from build123d import *

# Parameters (mm, degrees)
F1_FACE_R   = 15
F1_FACE_R_2 = 7
F2_DEPTH    = 5
F4_DEPTH    = 20


with BuildPart() as f1:
    # F0 (on Front) → F1 (revolve)
    with BuildSketch(Plane.XZ):
        Polygon((7, 27), (4, 27), (4, 8), (3, 8), (3, 4.470672), (4, 3.561659), (4, 0), (4, -1), (0, -1), (0, -25), (15, -25), (15, 27), (15, 30), (7, 30), align=None)
    revolve(axis=Axis((0, 0, -12.5), (0, 0, 1)))

    # F1_face (on face) → F2 (join)
    with BuildSketch(Plane.XY.offset(30)):
        Circle(F1_FACE_R)
        Circle(F1_FACE_R_2, mode=Mode.SUBTRACT)
    extrude(amount=F2_DEPTH)

    # F3 (on Front) → F4 (cut, symmetric)
    with BuildSketch(Plane.XZ):
        with BuildLine():
            Line((10.994077, 35.048041), (-10.997782, 35.048041))
            ThreePointArc((-10.997782, 35.048041), (-0.001852, 30), (10.994077, 35.048041))
        make_face()
    extrude(amount=F4_DEPTH, both=True, mode=Mode.SUBTRACT)


solid = f1.part
Work out the finished part from the listing and answer in its coordinate system (mm). A direction names the side the tool comes from. Coordinates: 2 decimals unless noted, no trailing zeros. Loops run counter-clockwise (first coordinate to the right, second up) from the corner with the lowest first, then second, coordinate; pieces in that order, holes last. Notation, with made-up numbers: M 52.5,89 L 70.5,89 A22 cw 70.5,118 Z; hole C 15,52.25 d10. An arc over 180 degrees is marked long. Answer in a Markdown table with one row per item. Add a question column.
1. Find section B-B, the plane x = 6. Write down the section's boundary in (y, z), then the cut area to 3 significant figures.
2. Find section C-C, the plane y = 5. Write down the section's boundary in (x, z).
3. Find section D-D, the plane z = -4. Write down the section's boundary in (x, y), then the cut area to 3 significant figures.
4. Consider L1, parallel to Y at x = 0, z = 1.1; L2, parallel to X at y = 0, z = 28.8; L3, parallel to Z at x = -6.5, y = -1.5. Determine where each line is inside the solid, lowest interval first.
5. Find section A-A, the plane z = 29. Write down the section's boundary in (x, y).
6. A tool of negligible diameter and unlimited length cuts with its end or side. For faces 1 (the cylindrical face through (-2.915, -6.877, 30.296)), 2 (the flat face through (3, -3, 27)), 3 (the cylindrical face through (-0.867, -3.905, 1.249)), from which of +Z, -Z, +X, -X, +Y, -Y can it reach the whole face along a straight path? Write none if from no direction.
7. The mould has two halves that part along Z. Classify faces 4 (the flat face through (1, 3, 8)), 5 (the cylindrical face through (-0.867, -3.905, 17.367)), 6 (the flat face through (0, 0, -1)): pulls with the +Z half, pulls with the -Z half, needs draft (parallel to the pull), parting line crosses it, or undercut.
8. Flat-ended cylindrical pins translate along their axes: P1, Ø8, axis at x = -8.5, y = -2.5, coming from the +Z side; P2, Ø5, axis at x = 7, z = -8.5, coming from the -Y side; P3, Ø5, axis at x = -11.5, z = -12.5, coming from the -Y side; P4, Ø15.5, axis at x = -1.5, y = 2, coming from the +Z side. Find the tip coordinate at first contact, or state that the pin passes through.
Reported:
| question | item | result |
|---|---|---|
| 1 | outline | M -13.75,-25 L 13.75,-25 L 13.75,31.3 L 3.61,31.3 L 3.61,27 L -3.61,27 L -3.61,31.3 L -13.75,31.3 Z |
| 1 | area | 1,520 mm^2 |
| 2 | outline | M -14.14,-25 L 14.14,-25 L 14.14,35 L 10.95,35 A14.5 cw 4.9,30.85 L 4.9,27 L -4.9,27 L -4.9,30.85 A14.5 cw -10.96,35 L -14.14,35 Z |
| 3 | outline | C 0,0 d30 |
| 3 | area | 707 mm^2 |
| 4 | L1 | y = -15 to -4, 4 to 15 |
| 4 | L2 | x = -15 to -7, 7 to 15 |
| 4 | L3 | z = -25 to 27 |
| 5 | outline | C 0,0 d30; hole C 0,0 d14 |
| 6 | face 1 | +Z, +Y, -Y |
| 6 | face 2 | +Z |
| 6 | face 3 | none |
| 7 | face 4 | pulls with the +Z half |
| 7 | face 5 | needs draft |
| 7 | face 6 | undercut |
| 8 | P1 | stops at z = 35 |
| 8 | P2 | stops at y = -14.31 |
| 8 | P3 | stops at y = -12 |
| 8 | P4 | stops at z = 33.33 |
